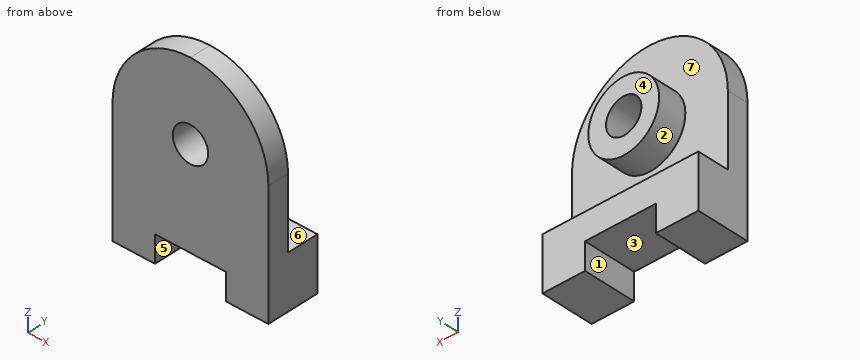
```python
from build123d import *

# Parameters (mm, degrees)
F1_DEPTH = 30
F2_DEPTH = 12
F3_DEPTH = 28


with BuildPart() as f1:
    # F0 (on Front) → F1 (new body)
    with BuildSketch(Plane.XZ):
        Polygon((-36.498324, -29.017857), (-80.498324, -29.017857), (-80.498324, -59.017857), (-56.498324, -59.017857), (-56.498324, -44.017857), (-36.498324, -44.017857), (-16.498324, -44.017857), (-16.498324, -59.017857), (7.501676, -59.017857), (7.501676, -29.017857), align=None)
    extrude(amount=-F1_DEPTH)

    # F0 (on Front) → F2 (join)
    with BuildSketch(Plane.XZ):
        with BuildLine():
            ThreePointArc((7.501676, 10.982143), (-5.385626, 42.094841), (-36.498324, 54.982143))
            ThreePointArc((-36.498324, 54.982143), (-67.611023, 42.094841), (-80.498324, 10.982143))
            Line((-80.498324, 10.982143), (-80.498324, -29.017857))
            Line((-80.498324, -29.017857), (-36.498324, -29.017857))
            Line((-36.498324, -29.017857), (7.501676, -29.017857))
            Line((7.501676, -29.017857), (7.501676, 10.982143))
        make_face()
        with BuildLine():
            ThreePointArc((-36.498324, -9.017857), (-56.498324, 10.982143), (-36.498324, 30.982143))
            ThreePointArc((-36.498324, 30.982143), (-16.498324, 10.982143), (-36.498324, -9.017857))
        make_face(mode=Mode.SUBTRACT)
    extrude(amount=-F2_DEPTH)

    # F0 (on Front) → F3 (join)
    with BuildSketch(Plane.XZ):
        with BuildLine():
            ThreePointArc((-36.498324, -9.017857), (-16.498324, 10.982143), (-36.498324, 30.982143))
            ThreePointArc((-36.498324, 30.982143), (-56.498324, 10.982143), (-36.498324, -9.017857))
        make_face()
        with BuildLine():
            ThreePointArc((-36.498324, 0.982143), (-46.498324, 10.982143), (-36.498324, 20.982143))
            ThreePointArc((-36.498324, 20.982143), (-26.498324, 10.982143), (-36.498324, 0.982143))
        make_face(mode=Mode.SUBTRACT)
    extrude(amount=-F3_DEPTH)


solid = f1.part
```
Geometry check sheet. Reference: the model listing, model coordinates, mm. Face numbers are marked on the shaded views. A direction names the side the tool comes from. Give positions to 0.01 mm unless a question says otherwise; leave off trailing zeros. Loops run counter-clockwise (first coordinate to the right, second up) from the corner with the lowest first, then second, coordinate; pieces in that order, holes last. Notation, with made-up numbers: M -29,84.5 L -4,84.5 A5 cw -4,91.5 Z; hole C -36.5,58.25 d5. An arc over 180 degrees is marked long. Answer as CSV lines item,"result".
Item 1: Access from +Z, -Z, +X, -X, +Y, -Y to the whole of each face (thin tool, end or side, straight path). Record for the marked faces 4, 5, 6 and 7.
Values:
face 4,"+Z, +X, -X, +Y"
face 5,"-Z, +Y, -Y"
face 6,"+X, -X, +Y"
face 7,"+Y"
Item 2: Release check for a two-part mould opening along Z. For the marked faces 1, 2 and 3 record: pulls with the +Z half, pulls with the -Z half, needs draft (parallel to the pull), parting line crosses it, or undercut.
Values:
face 1,"needs draft"
face 2,"undercut"
face 3,"pulls with the -Z half"
Item 3: Cross-section at C-C on x = -32. Record the cut outline in (y, z).
Values:
outline,"M 0,-44.02 L 30,-44.02 L 30,-29.02 L 12,-29.02 L 12,-8.51 L 28,-8.51 L 28,2.05 L 0,2.05 Z; M 0,19.91 L 28,19.91 L 28,30.47 L 12,30.47 L 12,54.75 L 0,54.75 Z"
Item 4: Cross-section at B-B on y = 3.75. Record the cut outline in (x, z), and give its area (3 significant figures).
Values:
outline,"M -80.5,-59.02 L -56.5,-59.02 L -56.5,-44.02 L -16.5,-44.02 L -16.5,-59.02 L 7.5,-59.02 L 7.5,10.98 A44 ccw -36.5,54.98 A44 ccw -80.5,10.98 Z; hole C -36.5,10.98 d20"
area,"8,290 mm²"
Item 5: Material ranges on line 1 (X direction, y = 13, z = -53); line 2 (Z direction, x = -36.5, y = 7.75); line 3 (Y direction, x = -57, z = -16), recorded low to high.
Values:
line 1,"x = -80.5 to -56.5, -16.5 to 7.5"
line 2,"z = -44.02 to 0.98, 20.98 to 54.98"
line 3,"y = 0 to 12"
Item 6: Cross-section at D-D on z = 29.5. Record the cut outline in (x, y), and give its area (3 significant figures).
Values:
outline,"M -76.41,0 L 3.42,0 L 3.42,12 L -28.94,12 L -28.94,28 L -44.05,28 L -44.05,12 L -76.41,12 Z"
area,"1,200 mm²"
Item 7: Cross-section at A-A on y = 14.5. Record the cut outline in (x, z), and give its area (3 significant figures).
Values:
outline,"M -80.5,-59.02 L -56.5,-59.02 L -56.5,-44.02 L -16.5,-44.02 L -16.5,-59.02 L 7.5,-59.02 L 7.5,-29.02 L -80.5,-29.02 Z; C -36.5,10.98 d40; hole C -36.5,10.98 d20"
area,"2,980 mm²"
Item 8: Depth check by flat-ended pin: P1, Ø12, axis at x = -37.5, z = 5, coming from the +Y side; P2, Ø9, axis at x = -53, y = 22, coming from the +Z side; P3, Ø10, axis at x = -17.5, y = 14.5, coming from the +Z side. Enter the tip coordinate at first touch or a pass-through.
Values:
P1,"stops at y = 28"
P2,"stops at z = 26.98"
P3,"stops at z = 52.47"
